Work out the finished part from the listing and answer in its coordinate system (mm). A direction names the side the tool comes from. Coordinates: 2 decimals unless noted, no trailing zeros. Order: outer loops, then holes, each group sorted by start corner. A loop starts at its lowest first (then second) coordinate and runs counter-clockwise, first axis right, second up. Notation, with made-up numbers: M 85.5,79 L 91.5,79 A12 ccw 91.5,96 Z; hole C 57.5,54.5 d3. An arc over 180 degrees is marked long. Use a Markdown table: item, result.
from build123d import *
from build123d.topology import SkipClean

# Parameters (mm, degrees)
SKETCH1_R             = 42.5
SKETCH1_R_2           = 14
SKETCH1_R_3           = 1.5
BOSS_EXTRUDE1_DEPTH   = 25
BOSS_EXTRUDE2_START   = 2
SKETCH2_R             = 14
SKETCH2_R_2           = 1.5
BOSS_EXTRUDE2_DEPTH   = 2
M4_TAPPED_HOLE1_D     = 3.3
M4_TAPPED_HOLE1_DEPTH = 5
M4_TAPPED_HOLE1_TIP   = 0.991420021


with BuildPart() as part:
    # Sketch1 → Boss-Extrude1 (new body)
    # profile 1 of 2: a face of its own
    with BuildSketch(Plane.XY):
        Circle(SKETCH1_R)
        Circle(SKETCH1_R_2, mode=Mode.SUBTRACT)
    # profile 2 of 2: a face of its own
    with BuildSketch(Plane.XY):
        Circle(SKETCH1_R_2)
        with Locations((-8.660254038, 5)):
            Circle(SKETCH1_R_3, mode=Mode.SUBTRACT)
        with Locations((-8.660254038, -5)):
            Circle(SKETCH1_R_3, mode=Mode.SUBTRACT)
        with Locations((0, -10)):
            Circle(SKETCH1_R_3, mode=Mode.SUBTRACT)
        with Locations((8.660254038, -5)):
            Circle(SKETCH1_R_3, mode=Mode.SUBTRACT)
        with Locations((8.660254038, 5)):
            Circle(SKETCH1_R_3, mode=Mode.SUBTRACT)
        with Locations((0, 10)):
            Circle(SKETCH1_R_3, mode=Mode.SUBTRACT)
    extrude(amount=BOSS_EXTRUDE1_DEPTH)

    # Sketch2 → Boss-Extrude2 (add)
    with SkipClean():  # the faces are left unmerged after this step: merging them gives an invalid solid
        with BuildSketch(Plane(origin=(0, 0, 0), x_dir=(-1, 0, 0), z_dir=(0, 0, -1)).offset(BOSS_EXTRUDE2_START)):
            with Locations(Location((0, 0, 0), (0, 0, 180))):
                Circle(SKETCH2_R)
            with Locations((0, 10)):
                Circle(SKETCH2_R_2, mode=Mode.SUBTRACT)
            with Locations((8.660254038, 5)):
                Circle(SKETCH2_R_2, mode=Mode.SUBTRACT)
            with Locations((8.660254038, -5)):
                Circle(SKETCH2_R_2, mode=Mode.SUBTRACT)
            with Locations((0, -10)):
                Circle(SKETCH2_R_2, mode=Mode.SUBTRACT)
            with Locations((-8.660254038, -5)):
                Circle(SKETCH2_R_2, mode=Mode.SUBTRACT)
            with Locations((-8.660254038, 5)):
                Circle(SKETCH2_R_2, mode=Mode.SUBTRACT)
        extrude(amount=-BOSS_EXTRUDE2_DEPTH)

    # M4 Tapped Hole1
    with Locations(Plane.XY.offset(25)):
        with Locations((0, 0)):
            Hole(M4_TAPPED_HOLE1_D / 2, depth=M4_TAPPED_HOLE1_DEPTH)
            with Locations((0, 0, -(M4_TAPPED_HOLE1_DEPTH + M4_TAPPED_HOLE1_TIP / 2))):  # 118° drill point
                Cone(0, M4_TAPPED_HOLE1_D / 2, M4_TAPPED_HOLE1_TIP, mode=Mode.SUBTRACT)


solid = part.part
1. Section D-D on x = -19.5 is taken. Determine the outline of the cut face in (y, z).
Answers below:
| item | result |
|---|---|
| outline | M -37.76,0 L 37.76,0 L 37.76,25 L -37.76,25 Z |
2. Find the intervals of material crossed by probe 1 along Y at (x, z) = (0, -0.4); probe 2 along X at (y, z) = (5, 17.5); probe 3 along Y at (x, z) = (10, 7), in increasing order.
Answers below:
| item | result |
|---|---|
| probe 1 | -14 to -11.5, -8.5 to 8.5, 11.5 to 14 |
| probe 2 | -42.2 to -10.16, -7.16 to 7.16, 10.16 to 42.2 |
| probe 3 | -41.31 to -5.67, -4.33 to 4.33, 5.67 to 41.31 |
3. Section C-C on x = 26.5 is taken. Determine the outline of the cut face in (y, z), then the cut area to 3 significant figures.
Answers below:
| item | result |
|---|---|
| outline | M -33.23,0 L 33.23,0 L 33.23,25 L -33.23,25 Z |
| area | 1,660 mm² |
4. Flat-ended cylindrical pins translate along their axes: P1, Ø4, axis at x = 28, y = 9.5, coming from the -Z side; P2, Ø2.5, axis at x = 8.66, y = 5, coming from the -Z side; P3, Ø3, axis at x = -25, z = 1.5, coming from the -Y side; P4, Ø2, axis at x = -29, z = 10.5, coming from the +Y side. Find the tip coordinate at first contact, or state that the pin passes through.
Answers below:
| item | result |
|---|---|
| P1 | z = 0 |
| P2 | through |
| P3 | y = -35.41 |
| P4 | y = 31.97 |
5. Section A-A on z = 11.75 is taken. Determine the outline of the cut face in (x, y), then the cut area to 3 significant figures.
Answers below:
| item | result |
|---|---|
| outline | C 0,0 d85; hole C -8.66,-5 d3; hole C -8.66,5 d3; hole C 0,-10 d3; hole C 0,10 d3; hole C 8.66,-5 d3; hole C 8.66,5 d3 |
| area | 5,630 mm² |
6. For a pull along Y with two mould halves and no side action, classify faces 4 (the face through (-33.727, -25.861, 12.325)), 5 (the face through (-0.1, -0.3, 19.2)), 6 (the face through (-10.04, 10.04, 0)) as +Y half, -Y half, draft (parallel to the pull), parting line (faces both ways), or undercut.
Answers below:
| item | result |
|---|---|
| face 4 | parting line |
| face 5 | undercut |
| face 6 | draft |
7. For faces 1 (the face through (12.932, 5.362, -1.014)), 2 (the face through (9, 1, 25)), 3 (the face through (1.216, 1.115, 22.465)), determine the directions among +Z, -Z, +X, -X, +Y, -Y from which every point of the face is accessible in a straight line to the end or side of a thin tool.
Answers below:
| item | result |
|---|---|
| face 1 | -Z |
| face 2 | +Z, +X, -X, +Y, -Y |
| face 3 | +Z |
8. Section B-B on y = -5 is taken. Determine the outline of the cut face in (x, z), then the cut area to 3 significant figures.
Answers below:
| item | result |
|---|---|
| outline | M -42.2,0 L -13.08,0 L -13.08,-2 L -10.16,-2 L -10.16,25 L -42.2,25 Z; M -7.16,-2 L 7.16,-2 L 7.16,25 L -7.16,25 Z; M 10.16,-2 L 13.08,-2 L 13.08,0 L 42.2,0 L 42.2,25 L 10.16,25 Z |
| area | 2,000 mm² |
